Here's the drawing with two shaded views (mm, measured from the low corner). I have some questions. A direction names the side the tool comes from. Give positions to 0.01 mm unless a question says otherwise; leave off trailing zeros. Loops run counter-clockwise (first coordinate to the right, second up) from the corner with the lowest first, then second, coordinate; pieces in that order, holes last. Notation, with made-up numbers: M 40.25,35.5 L 59.25,35.5 A15 ccw 59.25,54.5 Z; hole C -9,15.5 d11. An arc over 180 degrees is marked long. Use CSV: the item, a comma, the result in double quotes.
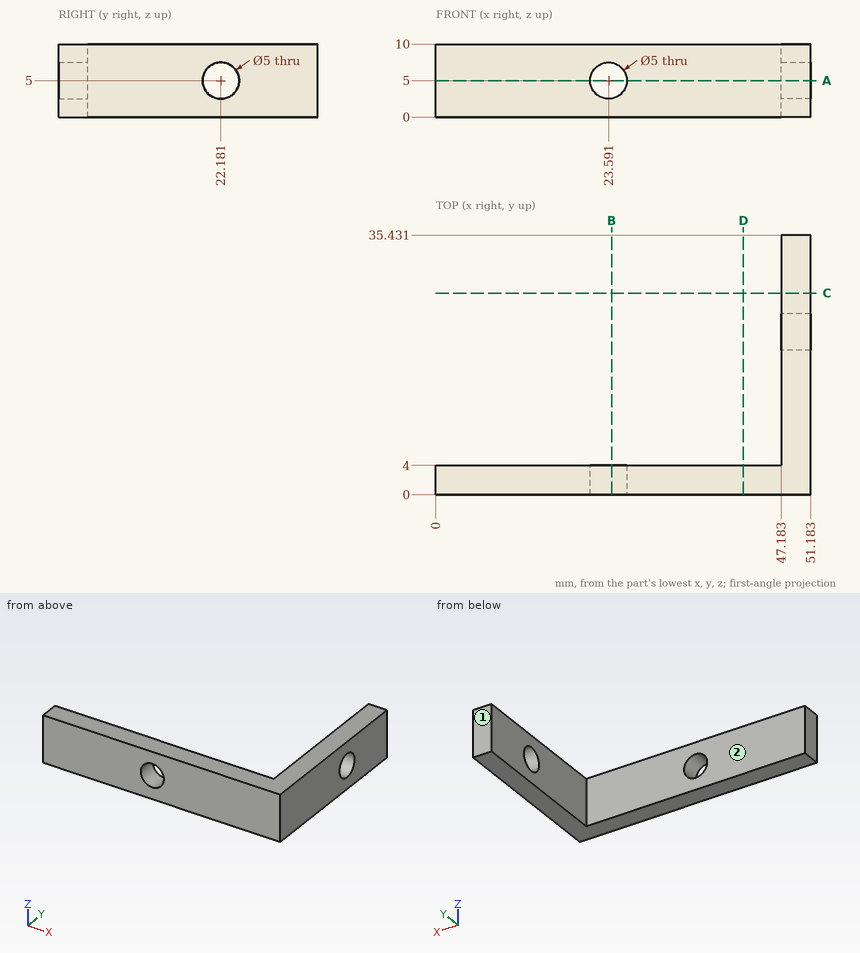
1. I want a section at C-C, the plane y = 27.5. List the corners of the cut face in (x, z) for me, then the cut area to 3 significant figures.
Outcome:
outline,"M 47.18,0 L 51.18,0 L 51.18,10 L 47.18,10 Z"
area,"40.0 mm2"
2. I want a section at B-B, the plane x = 24. List the corners of the cut face in (y, z) for me.
Outcome:
outline,"M 0,0 L 4,0 L 4,2.53 L 0,2.53 Z; M 0,7.47 L 4,7.47 L 4,10 L 0,10 Z"
3. I want a section at D-D, the plane x = 42. List the corners of the cut face in (y, z) for me, then the cut area to 3 significant figures.
Outcome:
outline,"M 0,0 L 4,0 L 4,10 L 0,10 Z"
area,"40.0 mm2"
4. Please list where these lines run through material, in increasing order: line 1 (X direction, y = 27, z = 8.75); line 2 (Y direction, x = 48.45, z = 5); line 3 (Y direction, x = 35, z = 4).
Outcome:
line 1,"47.18 to 51.18"
line 2,"0 to 19.68, 24.68 to 35.43"
line 3,"0 to 4"
5. Which directions (+Z, -Z, +X, -X, +Y, -Y) give clear straight access to the entire face, cutting with the end or side of a thin tool? Please do the marked faces 1 and 2.
Outcome:
face 1,"+Z, -Z, +X, -X, +Y"
face 2,"+Z, -Z, -X, +Y"
6. I'm going to push flat-ended pins straight in: pin 1 Ø3 at (x, z) = (8.5, 1) entering from +Y; pin 2 Ø5 at (y, z) = (18, 5) entering from -X; pin 3 Ø4 at (x, z) = (23.59, 5) entering from -Y. Where does each tip first touch, or does it pass through?
Outcome:
pin 1,"y = 4"
pin 2,"x = 47.18"
pin 3,"through"
7. I want a section at A-A, the plane z = 5. List the corners of the cut face in (x, y) for me.
Outcome:
outline,"M 0,0 L 21.09,0 L 21.09,4 L 0,4 Z; M 26.09,0 L 51.18,0 L 51.18,19.68 L 47.18,19.68 L 47.18,4 L 26.09,4 Z; M 47.18,24.68 L 51.18,24.68 L 51.18,35.43 L 47.18,35.43 Z"
